Source: CAD feature listing. Evaluate the final solid. Frame: model axes, mm. A direction names the side the tool comes from. Round coordinates to 2 decimals unless told otherwise and drop trailing zeros. Loops run counter-clockwise (first coordinate to the right, second up) from the corner with the lowest first, then second, coordinate; pieces in that order, holes last. Notation, with made-up numbers: (-23, 64.5) - (15, 64.5) arc R14 ccw to (15, 79.5) - close; hole circle Ø7 at (44, 22.5). An arc over 180 degrees is marked (long way). Write item = value, one per line. Start each with the question number.
from build123d import *

# Parameters (mm, degrees)
F1_DEPTH      = 52.07
F1_DEPTH_BACK = 52.07
F2_W          = 48.26
F2_H          = 3.175
F3_DEPTH      = 104.14
F4_W          = 104.14
F4_H          = 13.335
F5_DEPTH      = 3.175
F6_R          = 5.08
F7_DEPTH      = 3.175
F8_R          = 6.35
F9_DEPTH      = 51.435


with BuildPart() as f1:
    # F0 (on Right) → F1 (new body, two sides)
    with BuildSketch(Plane.YZ) as f1_sk:
        Polygon((29.21, 0), (29.21, 47.3075), (0, 47.3075), (-25.4, 16.51), (-25.4, 0), (-25.4, -16.51), (0, -47.3075), (29.21, -47.3075), align=None)
        Polygon((-22.225, 0), (-22.225, 3.175), (-22.225, 15.369625), (1.496958, 44.1325), (26.035, 44.1325), (26.035, 3.175), (26.035, 0), (26.035, -3.175), (26.035, -44.1325), (1.496958, -44.1325), (-22.225, -15.369625), (-22.225, -3.175), align=None, mode=Mode.SUBTRACT)
    extrude(amount=F1_DEPTH)
    extrude(f1_sk.sketch, amount=-F1_DEPTH_BACK)

    # F2 (on face) → F3 (join, through all)
    with BuildSketch(Plane.YZ.offset(52.07)):
        with Locations((1.905, 0)):
            Rectangle(F2_W, F2_H)
    extrude(amount=-F3_DEPTH)

    # F4 (on face) → F5 (join)
    with BuildSketch(Plane(origin=(0, 29.21, 0), x_dir=(-1, 0, 0), z_dir=(0, 1, 0))):
        with Locations((0, 53.975)):
            Rectangle(F4_W, F4_H)
        with Locations((0, -53.975)):
            Rectangle(F4_W, F4_H)
    extrude(amount=-F5_DEPTH)

    # F6 (on face) → F7 (cut, through all)
    with BuildSketch(Plane.XZ.offset(-26.035)):
        with Locations((-45.339, 53.975)):
            Circle(F6_R)
        with Locations((45.339, 53.975)):
            Circle(F6_R)
        with Locations((45.339, -53.975)):
            Circle(F6_R)
        with Locations((-45.339, -53.975)):
            Circle(F6_R)
    extrude(amount=-F7_DEPTH, mode=Mode.SUBTRACT)

    # F8 (on face) → F9 (cut, through all)
    with BuildSketch(Plane.XZ.offset(25.4)):
        with Locations((-31.75, 31.90875)):
            Circle(F8_R)
        with Locations((31.75, 31.90875)):
            Circle(F8_R)
        with Locations((31.75, -31.90875)):
            Circle(F8_R)
        with Locations((-31.75, -31.90875)):
            Circle(F8_R)
    extrude(amount=-F9_DEPTH, mode=Mode.SUBTRACT)


solid = f1.part
(1) Access query for faces 5 (the face through (1, 14, 44.132)), 6 (the face through (1, 13, 47.308)), 7 (the face through (-25.433, -10.676, -31.264)), 8 (the face through (1, 26.035, -54)). Directions: +Z, -Z, +X, -X, +Y, -Y. A direction counts if a zero-diameter tool reaches every point of the face in a straight line with its end or side. Return the directions, or none.
(2) Material intervals for line 1 along Z through (x, y) = (-25.5, 24); line 2 along Z through (x, y) = (-27.5, -21.5); line 3 along Y through (x, z) = (-29.5, -12.5) (3 decimals), sorted ascending. Write a range as from..to.
(3) Cut plane A-A (y = 6.5). Output: boundary loops of the cut face in (x, z).
(4) Mould query, pull axis Y, two halves, no side actions, for faces 1 (the face through (50, 28, -56)), 2 (the face through (1, 26.035, -23)), 3 (the face through (1, -25.4, 0)), 4 (the face through (0.73, -10.53, 29.55)). Classes: +Y half, -Y half, draft (parallel to the pull), parting line (faces both ways), or undercut.
(5) Cut plane C-C (x = 1). Output: boundary loops of the cut face in (y, z) (1 decimal).
(6) Cut plane D-D (z = 28). Output: boundary loops of the cut face in (x, y) (3 decimals).
(7) Pin query (flat end, axial travel): P1, Ø4, axis at y = 0, z = -5.5, coming from the -X side; P2, Ø24, axis at x = -0.5, y = 11, coming from the -Z side; P3, Ø10.5, axis at x = -0.5, z = 56, coming from the -Y side (3 decimals); P4, Ø14.5, axis at x = 31.75, z = 31.91, coming from the -Y side. Return the tip coordinate at first contact, or that it passes through.
(8) Cut plane B-B (z = 7.5). Output: boundary loops of the cut face in (x, y) (3 decimals), and give its area (3 significant figures).
Solution:
q1.face_5 = +X, -X
q1.face_6 = +Z, +X, -X, -Y
q1.face_7 = -Y
q1.face_8 = -Z, +X, -X, -Y
q2.line_1 = -47.31..-44.13, -1.59..1.59, 44.13..47.31
q2.line_2 = -21.24..-16.25, -1.59..1.59, 16.25..21.24
q2.line_3 = -25.4..-22.225, 26.035..29.21
q3.outline = (-52.07, -47.31) - (52.07, -47.31) - (52.07, -44.13) - (-52.07, -44.13) - close; (-52.07, -1.59) - (52.07, -1.59) - (52.07, 1.59) - (-52.07, 1.59) - close; (-52.07, 44.13) - (52.07, 44.13) - (52.07, 47.31) - (-52.07, 47.31) - close
q4.face_1 = draft
q4.face_2 = undercut
q4.face_3 = -Y half
q4.face_4 = undercut
q5.outline = (-25.4, -16.5) - (0, -47.3) - (26, -47.3) - (26, -60.6) - (29.2, -60.6) - (29.2, 60.6) - (26, 60.6) - (26, 47.3) - (0, 47.3) - (-25.4, 16.5) - close; hole (-22.2, -15.4) - (1.5, -44.1) - (26, -44.1) - (26, -1.6) - (-22.2, -1.6) - close; hole (-22.2, 1.6) - (26, 1.6) - (26, 44.1) - (1.5, 44.1) - (-22.2, 15.4) - close
q6.outline = (-52.07, -15.924) - (-36.754, -15.924) - (-36.754, -11.808) - (-52.07, -11.808) - close; (-52.07, 26.035) - (52.07, 26.035) - (52.07, 29.21) - (-52.07, 29.21) - close; (-26.746, -15.924) - (26.746, -15.924) - (26.746, -11.808) - (-26.746, -11.808) - close; (36.754, -15.924) - (52.07, -15.924) - (52.07, -11.808) - (36.754, -11.808) - close
q7.P1 = through
q7.P2 = -47.31
q7.P3 = 26.035
q7.P4 = -18.68
q8.outline = (-52.07, -25.4) - (52.07, -25.4) - (52.07, -22.225) - (-52.07, -22.225) - close; (-52.07, 26.035) - (52.07, 26.035) - (52.07, 29.21) - (-52.07, 29.21) - close
q8.area = 661 mm^2
